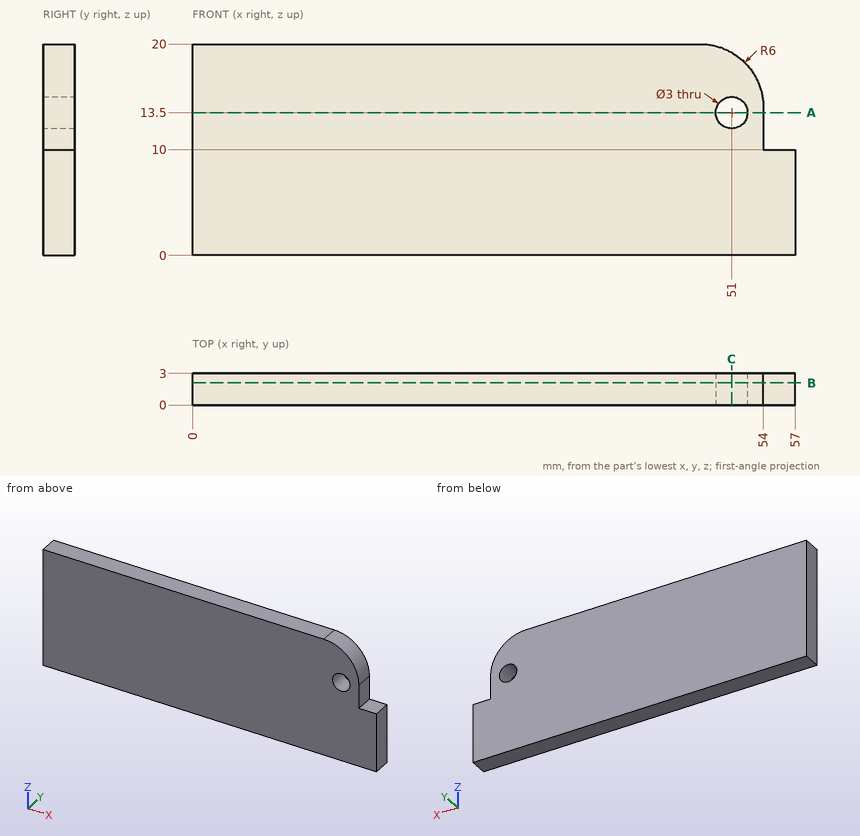
The drawing under review shows one solid part. Ordinate dimensions are in mm from its lowest x, y, z. Round coordinates to 2 decimals unless told otherwise and drop trailing zeros. Loops run counter-clockwise (first coordinate to the right, second up) from the corner with the lowest first, then second, coordinate; pieces in that order, holes last. Notation, with made-up numbers: (-31.75, 40.5) - (-19.75, 40.5) arc R34 ccw to (-19.75, 73.5) - close; hole circle Ø2 at (-0.5, 81). An arc over 180 degrees is marked (long way). One line per item, written item: value. Start each with the question number.
1) Consider section A-A on z = 13.5. Give the boundary of the cut face in (x, y).
2) To check wall thickness, follow L1, parallel to X at y = 0.7, z = 13.5; L2, parallel to X at y = 0.95, z = 12.5; L3, parallel to Z at x = 51.5, y = 0.9. State the ranges of each line that lie inside material, in increasing order. Write a range as from..to.
3) Consider section B-B on y = 2.1. Give the boundary of the cut face in (x, z).
4) Insertion check: pin 1 Ø0.9 at (x, y) = (55, 2) entering from +Z. The pin has a flat end and moves straight along its axis. Give the tip position at first contact, or say it passes through.
5) Consider section C-C on x = 51. Give the boundary of the cut face in (y, z), then the cut area to 3 significant figures.
Reported:
1. outline: (0, 0) - (49.5, 0) - (49.5, 3) - (0, 3) - close; (52.5, 0) - (54, 0) - (54, 3) - (52.5, 3) - close
2. L1: x = 0..49.5, 52.5..54
2. L2: x = 0..49.88, 52.12..54
2. L3: z = 0..12.09, 14.91..18.87
3. outline: (0, 0) - (57, 0) - (57, 10) - (54, 10) - (54, 14) arc R6 ccw to (48, 20) - (0, 20) - close; hole circle Ø3 at (51, 13.5)
4. pin 1: stops at z = 10
5. outline: (0, 0) - (3, 0) - (3, 12) - (0, 12) - close; (0, 15) - (3, 15) - (3, 19.2) - (0, 19.2) - close
5. area: 48.6 mm^2
